Model file for the job. Use its own axes, mm. A direction names the side the tool comes from. Round coordinates to 2 decimals unless told otherwise and drop trailing zeros. Loops run counter-clockwise (first coordinate to the right, second up) from the corner with the lowest first, then second, coordinate; pieces in that order, holes last. Notation, with made-up numbers: M 66.5,72.25 L 121.5,72.25 A14 cw 121.5,81.25 Z; hole C 56.5,12 d2. An arc over 180 degrees is marked long. Answer in a Markdown table with one row per item.
from build123d import *

# Parameters (mm, degrees)
F0_W     = 65.1002
F0_H     = 56.515
F0_R     = 20.3073
F1_DEPTH = 12.7
F2_W     = 15.875
F2_H     = 9.525
F3_DEPTH = 12.701
F4_R     = 2.5527
F5_DEPTH = 65.1012
F6_R     = 2.0193
F7_DEPTH = 49.2262


with BuildPart() as f1:
    # F0 (on Front) → F1 (new body)
    with BuildSketch(Plane.XZ):
        Rectangle(F0_W, F0_H)
        with Locations((0, 1.6002)):
            Circle(F0_R, mode=Mode.SUBTRACT)
    extrude(amount=F1_DEPTH)

    # F2 (on face) → F3 (cut, through all)
    with BuildSketch(Plane.XZ.offset(12.7)):
        with Locations((-24.6126, -23.495)):
            Rectangle(F2_W, F2_H)
        with Locations((24.6126, -23.495)):
            Rectangle(F2_W, F2_H)
    extrude(amount=-F3_DEPTH, mode=Mode.SUBTRACT)

    # F4 (on face) → F5 (cut, through all)
    with BuildSketch(Plane(origin=(-32.5501, 0, 0), x_dir=(0, -1, 0), z_dir=(-1, 0, 0))):
        with Locations((6.35, 17.4625)):
            Circle(F4_R)
        with Locations((6.35, -7.9375)):
            Circle(F4_R)
        with Locations((6.35, 4.7625)):
            Circle(F4_R)
    extrude(amount=-F5_DEPTH, mode=Mode.SUBTRACT)

    # F6 (on face) → F7 (cut, through all)
    with BuildSketch(Plane(origin=(-16.6751, 0, 0), x_dir=(0, -1, 0), z_dir=(-1, 0, 0))):
        with Locations((6.35, -23.495)):
            Circle(F6_R)
    extrude(amount=-F7_DEPTH, mode=Mode.SUBTRACT)


solid = f1.part
1. Saw through at C-C (y = -10). Write the cut outline in (x, z), and give its area (3 significant figures).
Verdict:
| item | result |
|---|---|
| outline | M -32.55,-18.73 L -16.68,-18.73 L -16.68,-28.26 L 16.68,-28.26 L 16.68,-18.73 L 32.55,-18.73 L 32.55,28.26 L -32.55,28.26 Z; hole C 0,1.6 d40.61 |
| area | 2,080 mm² |
2. Pin check, flat tips, straight feed: pin 1 (6.5 mm diameter, centred on x = -26, y = -6.5, fed in from -Z); pin 2 (4 mm diameter, centred on y = -6.35, z = -7.94, fed in from -X); pin 3 (5 mm diameter, centred on y = -3.5, z = -25, fed in from -X). Stop position of each tip, or through.
Verdict:
| item | result |
|---|---|
| pin 1 | stops at z = -18.73 |
| pin 2 | passes through |
| pin 3 | stops at x = -16.68 |
3. Saw through at D-D (x = 24.5). Write the cut outline in (y, z), and give its area (3 significant figures).
Verdict:
| item | result |
|---|---|
| outline | M -12.7,-18.73 L 0,-18.73 L 0,28.26 L -12.7,28.26 Z; hole C -6.35,-7.94 d5.11; hole C -6.35,4.76 d5.11; hole C -6.35,17.46 d5.11 |
| area | 535 mm² |
4. Mould opens along X. For faces 4 (the flat face through (-16.675, -6, -26)), 5 (the flat face through (32.55, -9, 4)), 6 (the cylindrical face through (-16.115, -6.261, -10.756)), 7 (the flat face through (0, -6, 28.258)) say: +X half, -X half, draft (parallel to the pull), parting line (faces both ways), or undercut.
Verdict:
| item | result |
|---|---|
| face 4 | -X half |
| face 5 | +X half |
| face 6 | undercut |
| face 7 | draft |
5. Saw through at A-A (x = 4.5). State how many separate pieces and enclosed holes the cut face has, and give its area (3 significant figures).
Verdict:
| item | result |
|---|---|
| separate pieces | 2 |
| enclosed holes | 1 |
| area | 202 mm² |
6. Tool access for faces 1 (the flat face through (25, -6, -18.732)), 2 (the flat face through (-25, -6, -18.732)), 3 (the cylindrical face through (-26.109, -7.722, 6.915)): list every direction of +Z, -Z, +X, -X, +Y, -Y with a clear straight run to the whole face (end or side of a thin tool).
Verdict:
| item | result |
|---|---|
| face 1 | -Z, +X, +Y, -Y |
| face 2 | -Z, -X, +Y, -Y |
| face 3 | +X, -X |
7. Saw through at B-B (z = 18.5). Write the cut outline in (x, y), and give its area (3 significant figures).
Verdict:
| item | result |
|---|---|
| outline | M -32.55,-12.7 L -11.26,-12.7 L -11.26,-8.68 L -32.55,-8.68 Z; M -32.55,-4.02 L -11.26,-4.02 L -11.26,0 L -32.55,0 Z; M 11.26,-12.7 L 32.55,-12.7 L 32.55,-8.68 L 11.26,-8.68 Z; M 11.26,-4.02 L 32.55,-4.02 L 32.55,0 L 11.26,0 Z |
| area | 342 mm² |
8. Wall check: probe 1 along Z at (x, y) = (27.5, -6.35); probe 2 along Z at (x, y) = (10, -6.5); probe 3 along Z at (x, y) = (-0.5, -2.75). Give the ranges that are in metal, low to high.
Verdict:
| item | result |
|---|---|
| probe 1 | z = -18.73 to -10.49, -5.38 to 2.21, 7.32 to 14.91, 20.02 to 28.26 |
| probe 2 | z = -28.26 to -25.51, -21.48 to -16.07, 20.01 to 28.26 |
| probe 3 | z = -28.26 to -18.7, 21.9 to 28.26 |
